CAD build for the part. Positions are in the model's coordinates, mm. Round coordinates to 2 decimals unless told otherwise and drop trailing zeros. Loops run counter-clockwise (first coordinate to the right, second up) from the corner with the lowest first, then second, coordinate; pieces in that order, holes last.
from build123d import *

# Parameters (mm, degrees)
BOSS_EXTRUDE1_DEPTH      = 500
BOSS_EXTRUDE1_DEPTH_BACK = 500
LPATTERN2_COUNT          = 17
LPATTERN2_PITCH          = 60
CHAMFER1_SIZE            = 0.5


with BuildPart() as part:
    # Sketch3 → Boss-Extrude1 (new, two sides: drawn at the far end of the back side and taken through both)
    with BuildSketch(Plane.XY.offset(-BOSS_EXTRUDE1_DEPTH_BACK)):
        with BuildLine():
            Line((3, 9), (-3, 9))
            Line((-3, 9), (-7.160036564, 9))
            Line((-7.160036564, 9), (-7.767930373, 8.392105714))
            ThreePointArc((-7.767930373, 8.392105714), (-8.344874488, 7.264307267), (-9.472673258, 6.687363783))
            Line((-9.472673258, 6.687363783), (-10, 6.160037041))
            Line((-10, 6.160037041), (-10, 4.82918644))
            Line((-10, 4.82918644), (-9.472673258, 4.314376637))
            ThreePointArc((-9.472673258, 4.314376637), (-8.341068744, 3.731631743), (-7.767930373, 2.595131504))
            Line((-7.767930373, 2.595131504), (-6.550048828, 1.379235268))
            Line((-6.550048828, 1.379235268), (-6.550048828, -1.550048828))
            Line((-6.550048828, -1.550048828), (-10, -4.999922752))
            Line((-10, -4.999922752), (-10, -8))
            Line((-10, -8), (-9, -9))
            Line((-9, -9), (0, -9))
            Line((0, -9), (9, -9))
            Line((9, -9), (10, -8))
            Line((10, -8), (10, -4.999922752))
            Line((10, -4.999922752), (6.550048828, -1.550048828))
            Line((6.550048828, -1.550048828), (6.550048828, 1.379235268))
            Line((6.550048828, 1.379235268), (7.767930373, 2.595131504))
            ThreePointArc((7.767930373, 2.595131504), (8.341068744, 3.731631743), (9.472673258, 4.314376637))
            Line((9.472673258, 4.314376637), (10, 4.82918644))
            Line((10, 4.82918644), (10, 6.160037041))
            Line((10, 6.160037041), (9.472673258, 6.687363783))
            ThreePointArc((9.472673258, 6.687363783), (8.344874488, 7.264307267), (7.767930373, 8.392105714))
            Line((7.767930373, 8.392105714), (7.160036564, 9))
            Line((7.160036564, 9), (3, 9))
        make_face()
    extrude(amount=BOSS_EXTRUDE1_DEPTH + BOSS_EXTRUDE1_DEPTH_BACK)

    # Sketch4 → Cut-Revolve1 (revolve, cut)
    with BuildSketch(Plane(origin=(0, 0, 0), x_dir=(0, 0, -1), z_dir=(1, 0, 0)), mode=Mode.PRIVATE) as cut_revolve1_sk:
        Polygon((-475.25, 9), (-480, 9), (-480, -9), (-477, -9), (-477, 0.5), (-475.25, 0.5), align=None)
    cut_revolve1 = revolve(cut_revolve1_sk.sketch.rotate(Axis((0, 9, 480), (0, -1, 0)), 180), axis=Axis((0, 9, 480), (0, -1, 0)), mode=Mode.SUBTRACT)

    # LPattern2: Cut-Revolve1 ×17
    with Locations(*[(0, 0, -i * LPATTERN2_PITCH) for i in range(1, LPATTERN2_COUNT)]):
        add(cut_revolve1, mode=Mode.SUBTRACT)

    # Chamfer1
    chamfer1_edges = [part.edges().sort_by_distance(p)[0] for p in [
        (-6.550048828, -0.08540678, 500),
        (-8.275024414, -3.27498579, 500),
        (-10, -6.499961376, 500),
        (-9.5, -8.5, 500),
        (0, -9, 500),
        (9.5, -8.5, 500),
        (10, -6.499961376, 500),
        (8.275024414, -3.27498579, 500),
        (6.550048828, -0.08540678, 500),
        (-8.341068744, 3.731631743, 500),
        (7.158989601, 1.987183386, 500),
        (8.341068744, 3.731631743, 500),
        (9.736336629, 4.571781538, 500),
        (-9.736336629, 4.571781538, -500),
        (-10, 5.49461174, -500),
        (10, 5.49461174, 500),
        (-9.736336629, 6.423700412, -500),
        (-7.463983469, 8.696052857, -500),
        (0, 9, -500),
        (7.463983469, 8.696052857, -500),
        (9.736336629, 6.423700412, -500),
        (10, 5.49461174, -500),
        (9.736336629, 6.423700412, 500),
        (9.736336629, 4.571781538, -500),
        (7.158989601, 1.987183386, -500),
        (6.550048828, -0.08540678, -500),
        (8.275024414, -3.27498579, -500),
        (10, -6.499961376, -500),
        (9.5, -8.5, -500),
        (0, -9, -500),
        (8.344874488, 7.264307267, 500),
        (-9.5, -8.5, -500),
        (-10, -6.499961376, -500),
        (-8.275024414, -3.27498579, -500),
        (-6.550048828, -0.08540678, -500),
        (-7.158989601, 1.987183386, -500),
        (-8.341068744, 3.731631743, -500),
        (-8.344874488, 7.264307267, -500),
        (8.344874488, 7.264307267, -500),
        (8.341068744, 3.731631743, -500),
        (7.463983469, 8.696052857, 500),
        (0, 9, 500),
        (-7.463983469, 8.696052857, 500),
        (-8.344874488, 7.264307267, 500),
        (-7.158989601, 1.987183386, 500),
        (-9.736336629, 6.423700412, 500),
        (-10, 5.49461174, 500),
        (-9.736336629, 4.571781538, 500),
    ]]
    chamfer(chamfer1_edges, length=CHAMFER1_SIZE)


solid = part.part
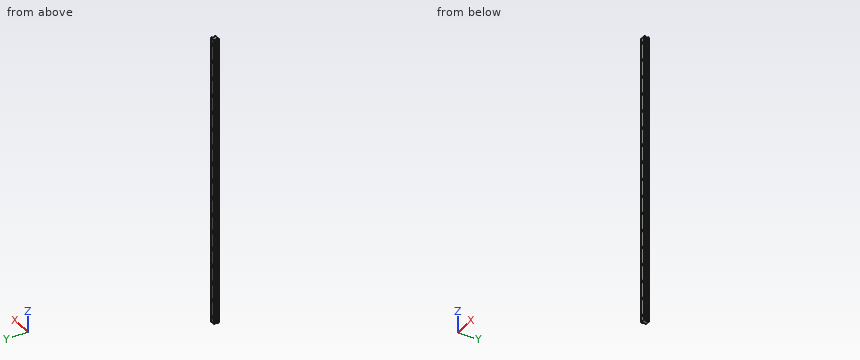
Item 1: Flat gauge pins, fed straight in: P1, Ø3.5, axis at x = 0, z = 480, coming from the +Y side; P2, Ø8, axis at x = 0, z = -480, coming from the +Y side; P3, Ø3, axis at y = 1.5, z = 352, coming from the +X side. Where does each tip first touch, or does it go through?
Verdict:
P1: passes through
P2: stops at y = 0.5
P3: stops at x = 7.87
Item 2: Wall check: L1, parallel to X at y = -5.75, z = 360; L2, parallel to X at y = -3.75, z = 420; L3, parallel to Y at x = 6.75, z = 196. Give the ranges that are in metal, low to high.
Verdict:
L1: x = -10 to -3, 3 to 10
L2: x = -8.75 to -3, 3 to 8.75
L3: y = -9 to -1.75, 1.58 to 9
Item 3: Cut at A-A (z = -89). List the corners of the cut face in (x, y), plus the area to 3 significant figures.
Verdict:
outline: (-10, -8) - (-9, -9) - (9, -9) - (10, -8) - (10, -5) - (6.55, -1.55) - (6.55, 1.38) - (7.77, 2.6) arc R2.06 cw to (9.47, 4.31) - (10, 4.83) - (10, 6.16) - (9.47, 6.69) arc R2.06 cw to (7.77, 8.39) - (7.16, 9) - (-7.16, 9) - (-7.77, 8.39) arc R2.06 cw to (-9.47, 6.69) - (-10, 6.16) - (-10, 4.83) - (-9.47, 4.31) arc R2.06 cw to (-7.77, 2.6) - (-6.55, 1.38) - (-6.55, -1.55) - (-10, -5) - close
area: 304 mm2
